Verification items for the finished model (mm, model axes). A direction names the side the tool comes from. Round coordinates to 2 decimals unless told otherwise and drop trailing zeros. Loops run counter-clockwise (first coordinate to the right, second up) from the corner with the lowest first, then second, coordinate; pieces in that order, holes last. Notation, with made-up numbers: M 70,82.25 L 103,82.25 A14 ccw 103,87.25 Z; hole C 85.25,69.5 d9. An arc over 180 degrees is marked long. Write item = value, one per line. Start each with the question number.
Autodesk Inventor part; units mm, degrees
ref_plane "Начальная плоскость" through (0, 0, 65.0657) normal (0, 0, 1) x (1, 0, 0)
ref_plane "Конечная плоскость" through (0, 0, 145) normal (0, 0, 1) x (1, 0, 0)
ref_plane "РабПлоскость8" through (18, 50.815, 145) normal (0, 0, 1) x (1, 0, 0)
ref_plane "Начальная плоскость" through (0, 0, 65.0657) normal (0, 0, 1) x (1, 0, 0)
ref_plane "Конечная плоскость" through (0, 0, 145) normal (0, 0, 1) x (1, 0, 0)
sketch "Эскиз" plane through (0, 0, 0) normal (0, 0, 1) x (1, 0, 0)
  line L0 (36, -32.5) -> (0, -32.5)
  line L1 (36, -32.5) -> (36, -28.696)
  line L2 (33.6994, -26.2039) -> (9.9215, -24.3017)
  line L3 (4.4, -18.3208) -> (4.4, 18.3208)
  line L4 (33.6994, 26.2039) -> (9.9215, 24.3017)
  line L5 (36, 28.696) -> (36, 32.5)
  line L6 (0, 32.5) -> (36, 32.5)
  line L7 (0, -32.5) -> (0, 32.5)
  arc A0 (4.4, -18.3208) -> (9.9215, -24.3017) centre (10.4, -18.3208) ccw
  arc A1 (9.9215, 24.3017) -> (4.4, 18.3208) centre (10.4, 18.3208) ccw
  arc A2 (36, -28.696) -> (33.6994, -26.2039) centre (33.5, -28.696) ccw
  arc A3 (33.6994, 26.2039) -> (36, 28.696) centre (33.5, 28.696) ccw
  line L8 (0, 45.5) -> (0, -45.5) construction
  line L9 (-7.2974, 0) -> (43.7847, 0) construction
  point P0 (36, -26.388)
  point P1 (4.4, -23.86)
  point P2 (4.4, 23.86)
  point P3 (36, 26.388)
  dimension "d3" = 36
  dimension "d5" = 4.4
  dimension "d7" = 65
  dimension "d9" = 8.64
  dimension "d11" = 8.64
  dimension "d13" = 6.112
  dimension "d15" = 6.112
  dimension "d22" = 6
  dimension "d23" = 2.5
  dimension "d24" = 32.5
  dimension "d25" = 0
extrude "Тело" add sketch "Эскиз" along normal up to surface (79.9343 mm away) from surface at 65.0657
sketch "Sketch3" plane through (0, 0, 0) normal (0, 0, 1) x (1, 0, 0)
  line L0 (0, 0) -> (10, 0)
ref_plane "Work Plane7" through (0, 0, 0) normal (0, -1, 0) x (1, 0, 0)
sketch "Sketch4" plane through (0, 0, 0) normal (0, -1, 0) x (1, 0, 0)
  line L0 (-2, 65.0657) -> (12, 65.0657)
  line L1 (-2, 145) -> (12, 145)
  dimension "d29" = 79.9343
ref_plane "РабПлоскость8" through (18, 50.815, 145) normal (0, 0, 1) x (1, 0, 0)
split "Разделение1" plane through (18, 50.815, 145) removes the side toward (0, 0, 1)
ref_plane "РабПлоскость9" through (18, -32.2683, 65.2966) normal (0, -0.0036, -1) x (1, 0, 0)
split "Разделение2" plane through (18, -32.2683, 65.2966) removes the side toward (0, -0.0036, -1)
equation "\"d3\" = b"
equation "\"d7\" = ParH"
equation "\"d22\" = R"
equation "\"d23\" = R1"
equation "\"d24\" = 0.5 * d7"
equation "\"d16\" = G_L"
equation "\"R1\" = 2.5"
equation "\"R\" = 6"
equation "\"t1\" = 4.4"
equation "\"t2\" = 7.2"
equation "\"ParH\" = 65"
equation "\"b\" = 36"
equation "\"msp_x1\" = 0.04 * b"
equation "\"msp_x2\" = -0.08 * t1 + 0.04 * b"
equation "\"G_L\" = d29"
equation "\"ex\" = 0"
equation "\"G_OFFSET_START\" = -65.06571"
equation "\"G_OFFSET_END\" = -65"
equation "\"d26\" = -G_OFFSET_START"
equation "\"d27\" = G_OFFSET_END + B_L"
properties part number "Швеллер 6.5U-79,93 ГОСТ 8240-97" material "Сталь, мягкая, сварочная"
1. Section check B-B, the plane x = 30. Enter the section's corners in (y, z).
2. Thickness scan on line 1 (X direction, y = -17, z = 134.5); line 2 (Y direction, x = 31, z = 114.5); line 3 (Y direction, x = 24, z = 122.5). Record the ranges inside material, lowest first.
3. Mould release check, pull along Y, two halves, no side actions. Record for faces 1 (the flat face through (36, 31, 104)), 2 (the flat face through (18, -32.5, 105)), 3 (the flat face through (21.977, 25.266, 104.484)): pulls with the +Y half, pulls with the -Y half, needs draft (parallel to the pull), parting line crosses it, or undercut.
4. Section check A-A, the plane z = 77. Enter the section's corners in (x, y), and give its area (3 significant figures).
5. Tool access check on faces 4 (the flat face through (18, 32.5, 104)), 5 (the cylindrical face through (6, -22.4, 104.6)). Record the directions out of +Z, -Z, +X, -X, +Y, -Y that give a thin tool (end or side, any length) a straight path to the whole face; none if there is none.
6. Section check D-D, the plane y = -4. Enter the section's corners in (x, z), and give its area (3 significant figures).
7. Section check C-C, the plane y = -19.5. Enter the section's corners in (x, z).
Computed values:
q1.outline = M -32.5,65.3 L -25.91,65.27 L -25.91,145 L -32.5,145 Z; M 25.91,65.09 L 31.87,65.07 L 32.5,65.07 L 32.5,145 L 25.91,145 Z
q2.line_1 = 0 to 4.4
q2.line_2 = -32.5 to -25.99, 25.99 to 32.5
q2.line_3 = -32.5 to -25.43, 25.43 to 32.5
q3.face_1 = needs draft
q3.face_2 = pulls with the -Y half
q3.face_3 = undercut
q4.outline = M 0,-32.5 L 36,-32.5 L 36,-28.7 A2.5 ccw 33.7,-26.2 L 9.92,-24.3 A6 cw 4.4,-18.32 L 4.4,18.32 A6 cw 9.92,24.3 L 33.7,26.2 A2.5 ccw 36,28.7 L 36,32.5 L 0,32.5 Z
q4.area = 763 mm2
q5.face_4 = +Z, -Z, +X, -X, +Y
q5.face_5 = +Z, -Z, +X
q6.outline = M 0,65.19 L 4.4,65.19 L 4.4,145 L 0,145 Z
q6.area = 351 mm2
q7.outline = M 0,65.25 L 4.52,65.25 L 4.52,145 L 0,145 Z
